```python
from build123d import *

# Parameters (mm, degrees)
SKETCH_1_W          = 55
SKETCH_1_H          = 65
SKETCH_1_R          = 1.5
EXTRUDE_1_DEPTH     = 1.5
CUT_EXTRUDE_1_DEPTH = 1.5
SKETCH_3_R          = 7.5
CUT_EXTRUDE_2_DEPTH = 43.599882629
FILLET_1_R          = 2
FILLET_2_R          = 1.5


with BuildPart() as part:
    # 草图1 → 凸台-拉伸1 (new body)
    with BuildSketch(Plane(origin=(0, 0, 0), x_dir=(1, 0, 0), z_dir=(0, 1, 0))):
        Rectangle(SKETCH_1_W, SKETCH_1_H)
        with Locations(Location((-25, 30, 0), (0, 0, 270))):
            Circle(SKETCH_1_R, mode=Mode.SUBTRACT)
        with Locations(Location((25, 30, 0), (0, 0, 270))):
            Circle(SKETCH_1_R, mode=Mode.SUBTRACT)
        with Locations(Location((25, -30, 0), (0, 0, 270))):
            Circle(SKETCH_1_R, mode=Mode.SUBTRACT)
        with Locations(Location((-25, -30, 0), (0, 0, 270))):
            Circle(SKETCH_1_R, mode=Mode.SUBTRACT)
    extrude(amount=EXTRUDE_1_DEPTH)

    # 草图2 → 切除-拉伸1 (cut)
    with BuildSketch(Plane(origin=(0, 1.5, 0), x_dir=(1, 0, 0), z_dir=(0, 1, 0))):
        with BuildLine():
            Line((-21.081475452, 23.202795796), (-6.939339828, 9.060660172))
            ThreePointArc((-6.939339828, 9.060660172), (-6.939339828, 6.939339828), (-9.060660172, 6.939339828))
            Line((-9.060660172, 6.939339828), (-23.202795796, 21.081475452))
            ThreePointArc((-23.202795796, 21.081475452), (-23.202795796, 23.202795796), (-21.081475452, 23.202795796))
        make_face()
        with BuildLine():
            Line((21.081475452, 23.202795796), (6.939339828, 9.060660172))
            ThreePointArc((6.939339828, 9.060660172), (6.939339828, 6.939339828), (9.060660172, 6.939339828))
            Line((9.060660172, 6.939339828), (23.202795796, 21.081475452))
            ThreePointArc((23.202795796, 21.081475452), (23.202795796, 23.202795796), (21.081475452, 23.202795796))
        make_face()
        with BuildLine():
            Line((23.202795796, -21.081475452), (9.060660172, -6.939339828))
            ThreePointArc((9.060660172, -6.939339828), (6.939339828, -6.939339828), (6.939339828, -9.060660172))
            Line((6.939339828, -9.060660172), (21.081475452, -23.202795796))
            ThreePointArc((21.081475452, -23.202795796), (23.202795796, -23.202795796), (23.202795796, -21.081475452))
        make_face()
        with BuildLine():
            Line((-21.081475452, -23.202795796), (-6.939339828, -9.060660172))
            ThreePointArc((-6.939339828, -9.060660172), (-6.939339828, -6.939339828), (-9.060660172, -6.939339828))
            Line((-9.060660172, -6.939339828), (-23.202795796, -21.081475452))
            ThreePointArc((-23.202795796, -21.081475452), (-23.202795796, -23.202795796), (-21.081475452, -23.202795796))
        make_face()
    extrude(amount=-CUT_EXTRUDE_1_DEPTH, mode=Mode.SUBTRACT)

    # 草图3 → 切除-拉伸2 (cut, through all)
    with BuildSketch(Plane(origin=(0, 1.5, 0), x_dir=(1, 0, 0), z_dir=(0, 1, 0))):
        with Locations(Location((0, 0, 0), (0, 0, 270))):
            Circle(SKETCH_3_R)
        Polygon((-22.5, 32.5), (0, 10), (22.5, 32.5), align=None)
        Polygon((-27.5, 17.5), (-10, 0), (-27.5, -17.5), align=None)
        Polygon((10, 0), (27.5, -17.5), (27.5, 17.5), align=None)
        Polygon((0, -10), (22.5, -32.5), (-22.5, -32.5), align=None)
    extrude(amount=-CUT_EXTRUDE_2_DEPTH, mode=Mode.SUBTRACT)

    # 圆角1
    fillet_1_edges = [part.edges().sort_by_distance(p)[0] for p in [
        (-10, 0.75, 0),
        (10, 0.75, 0),
        (0, 0.75, 10),
        (0, 0.75, -10),
    ]]
    fillet(fillet_1_edges, radius=FILLET_1_R)

    # 圆角2
    fillet_2_edges = [part.edges().sort_by_distance(p)[0] for p in [
        (-27.5, 0.75, 17.5),
        (-27.5, 0.75, -17.5),
        (27.5, 0.75, -17.5),
        (27.5, 0.75, 17.5),
        (-22.5, 0.75, 32.5),
        (22.5, 0.75, 32.5),
        (-22.5, 0.75, -32.5),
        (22.5, 0.75, -32.5),
        (27.5, 0.75, 32.5),
        (-27.5, 0.75, 32.5),
        (-27.5, 0.75, -32.5),
        (27.5, 0.75, -32.5),
    ]]
    fillet(fillet_2_edges, radius=FILLET_2_R)


solid = part.part
```
Here's how the part is built. I have some questions about the finished solid (model axes, mm). A direction names the side the tool comes from. Round coordinates to 2 decimals unless told otherwise and drop trailing zeros. Order: outer loops, then holes, each group sorted by start corner. A loop starts at its lowest first (then second) coordinate and runs counter-clockwise, first axis right, second up. Notation, with made-up numbers: (58, 29.25) -> (91, 29.25) arc R19 ccw to (91, 37.25) -> close; hole circle Ø1 at (61, 12). An arc over 180 degrees is marked (long way). Use a Markdown table: item, result. Add a question column.
(1) For pin 1 Ø2.5 at (x, z) = (-25, -30) entering from +Y, with a flat end and sliding along its axis, tell me the tip position at first contact or that it passes through.
(2) If we mould it in two halves opening along X, with no side actions, what happens to faces 1 (the face through (-27.5, 1, 25)), 2 (the face through (-6, 1.5, 7)), 3 (the face through (13.91, 0.76, 16.03)), 4 (the face through (6.92, 0.76, -6.96))? For each: released by +X, released by -X, zero draft, split by the parting line, or undercut.
(3) I need wall thicknesses on line 1 along X through (y, z) = (1.15, 15); line 2 along Z through (x, y) = (-18, 0.9); line 3 along Z through (x, y) = (23, 0.35). Which ranges of each line are inside material? Lowest first, please.
(4) Suppose I cut it at C-C, the plane z = 0. Please give me the cut outline in (x, y), and give its area (3 significant figures).
(5) Suppose I cut it at D-D, the plane x = 0. Please give me the cut outline in (y, z), and give its area (3 significant figures).
(6) Suppose I cut it at A-A, the plane x = -25. Please give me the cut outline in (y, z).
(7) For faces 5 (the face through (-19, 1, -9)), 6 (the face through (19, 1, -9)), 7 (the face through (-14.11, 0.76, 16.23)), 8 (the face through (12, 1, -22)), which set-ups out of +Z, -Z, +X, -X, +Y, -Y let a thin tool reach every point of the face, with its end or its side?
(8) Suppose I cut it at B-B, the plane z = 30. Please give me the cut outline in (x, y).
Verdict:
| question | item | result |
|---|---|---|
| 1 | pin 1 | through |
| 2 | face 1 | released by -X |
| 2 | face 2 | zero draft |
| 2 | face 3 | undercut |
| 2 | face 4 | undercut |
| 3 | line 1 | -25 to -17.12, -12.88 to -5, 5 to 12.88, 17.12 to 25 |
| 3 | line 2 | -28 to -20.12, -15.88 to -8, 8 to 15.88, 20.12 to 28 |
| 3 | line 3 | -32.5 to -23.37, -20.88 to -13, 13 to 20.88, 23.37 to 32.5 |
| 4 | outline | (-10.83, 0) -> (-7.5, 0) -> (-7.5, 1.5) -> (-10.83, 1.5) -> close; (7.5, 0) -> (10.83, 0) -> (10.83, 1.5) -> (7.5, 1.5) -> close |
| 4 | area | 9.99 mm2 |
| 5 | outline | (0, -10.83) -> (1.5, -10.83) -> (1.5, -7.5) -> (0, -7.5) -> close; (0, 7.5) -> (1.5, 7.5) -> (1.5, 10.83) -> (0, 10.83) -> close |
| 5 | area | 9.99 mm2 |
| 6 | outline | (0, -32.5) -> (1.5, -32.5) -> (1.5, -31.5) -> (0, -31.5) -> close; (0, -28.5) -> (1.5, -28.5) -> (1.5, -15) -> (0, -15) -> close; (0, 15) -> (1.5, 15) -> (1.5, 28.5) -> (0, 28.5) -> close; (0, 31.5) -> (1.5, 31.5) -> (1.5, 32.5) -> (0, 32.5) -> close |
| 7 | face 5 | -X, +Y, -Y |
| 7 | face 6 | +X, +Y, -Y |
| 7 | face 7 | +Y, -Y |
| 7 | face 8 | -Z, +Y, -Y |
| 8 | outline | (-27.5, 0) -> (-26.5, 0) -> (-26.5, 1.5) -> (-27.5, 1.5) -> close; (-23.5, 0) -> (-20, 0) -> (-20, 1.5) -> (-23.5, 1.5) -> close; (20, 0) -> (23.5, 0) -> (23.5, 1.5) -> (20, 1.5) -> close; (26.5, 0) -> (27.5, 0) -> (27.5, 1.5) -> (26.5, 1.5) -> close |
